Geometry: see drawing. Coordinates: mm, zero at the bounding-box minimum. A direction names the side the tool comes from. Round coordinates to 2 decimals unless told otherwise and drop trailing zeros. Write each loop counter-clockwise with the first axis right and the second up, starting at its lowest first coordinate (ties: lowest second). Pieces come first, ordered by that corner, then holes. Notation, with made-up numbers: (-1.75, -29) -> (21.25, -29) arc R16 cw to (21.25, -15) -> close; hole circle Ø5 at (11.5, -17.75). An arc over 180 degrees is marked (long way). Write item = value, one per line.
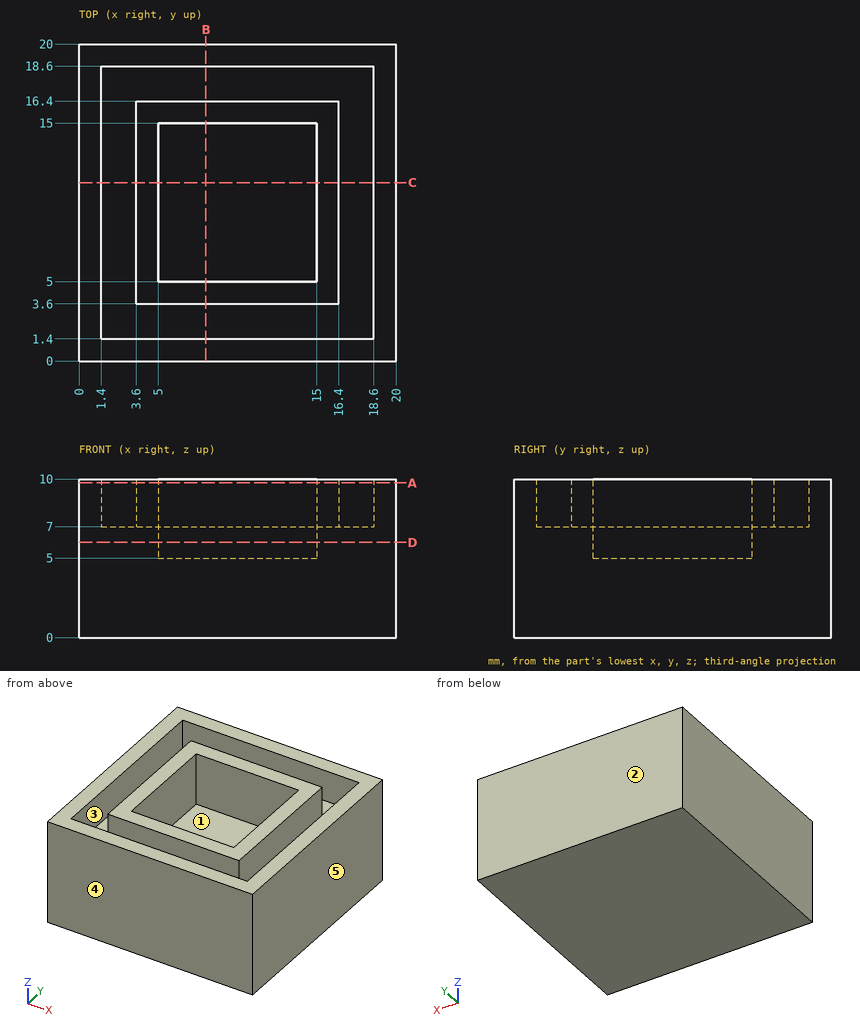
1) First-contact query: P1, Ø5, axis at x = 9, y = 9, coming from the +Z side. Flat tip, straight axial feed; report the tip coordinate or a pass-through.
Solutions:
P1 = 5
2) Cut plane B-B (x = 8). Return the cut outline in (y, z).
Solutions:
outline = (0, 0) -> (20, 0) -> (20, 10) -> (18.6, 10) -> (18.6, 7) -> (16.4, 7) -> (16.4, 10) -> (15, 10) -> (15, 5) -> (5, 5) -> (5, 10) -> (3.6, 10) -> (3.6, 7) -> (1.4, 7) -> (1.4, 10) -> (0, 10) -> close
3) Line query: L1, parallel to X at y = 14.5, z = 9.75; L2, parallel to X at y = 16.25, z = 7.5. Output: solid intervals per line, ascending. Write a range as from..to.
Solutions:
L1 = 0..1.4, 3.6..5, 15..16.4, 18.6..20
L2 = 0..1.4, 3.6..16.4, 18.6..20
4) Access query for the marked faces 1 and 2. Directions: +Z, -Z, +X, -X, +Y, -Y. A direction counts if a zero-diameter tool reaches every point of the face in a straight line with its end or side. Return the directions, or none.
Solutions:
face_1 = +Z
face_2 = +Z, -Z, +X, -X, +Y
5) Cut plane A-A (z = 9.75). Return the cut outline in (x, y), and give its area (3 significant figures).
Solutions:
outline = (0, 0) -> (20, 0) -> (20, 20) -> (0, 20) -> close; (3.6, 3.6) -> (16.4, 3.6) -> (16.4, 16.4) -> (3.6, 16.4) -> close; hole (1.4, 1.4) -> (18.6, 1.4) -> (18.6, 18.6) -> (1.4, 18.6) -> close; hole (5, 5) -> (15, 5) -> (15, 15) -> (5, 15) -> close
area = 168 mm^2
6) Cut plane D-D (z = 6). Return the cut outline in (x, y).
Solutions:
outline = (0, 0) -> (20, 0) -> (20, 20) -> (0, 20) -> close; hole (5, 5) -> (15, 5) -> (15, 15) -> (5, 15) -> close
7) Draft query along Y for the marked faces 3, 4 and 5. Return one class per face: +Y half, -Y half, draft (parallel to the pull), parting line (faces both ways), or undercut.
Solutions:
face_3 = undercut
face_4 = -Y half
face_5 = draft
